```python
from build123d import *

# Parameters (mm, degrees)
Y_KSEKLIK_EKSTR_ZYON1_DEPTH = 3
RADYUS1_R                   = 0.5
KES_EKSTR_ZYON2_REACH       = 38.886
IZIM6_W                     = 13
IZIM6_H                     = 2.5


with BuildPart() as part:
    # Çizim1 → Yükseklik-Ekstrüzyon1 (new body)
    with BuildSketch(Plane.XY):
        Polygon((10, 21.25), (30, 21.25), (30, 6.25), (10, 6.25), (10, -18.75), (-10, -18.75), (-10, 21.25), align=None)
    extrude(amount=Y_KSEKLIK_EKSTR_ZYON1_DEPTH)

    # Radyus1
    radyus1_edges = [part.edges().sort_by_distance(p)[0] for p in [
        (-10, 21.25, 1.5),
        (30, 21.25, 1.5),
        (30, 6.25, 1.5),
        (10, -18.75, 1.5),
        (-10, -18.75, 1.5),
    ]]
    fillet(radyus1_edges, radius=RADYUS1_R)

    # Çizim6 → Kes-Ekstrüzyon2 (cut, up to next)
    with BuildSketch(Plane(origin=(0, 0, 0), x_dir=(-1, 0, 0), z_dir=(0, 0, -1)), mode=Mode.PRIVATE) as kes_ekstr_zyon2_sk1:
        with Locations((-17.130228212, 18)):
            Rectangle(IZIM6_W, IZIM6_H)
    kes_ekstr_zyon2_tool1 = extrude(kes_ekstr_zyon2_sk1.sketch, amount=-KES_EKSTR_ZYON2_REACH, mode=Mode.PRIVATE) & part.part
    add(kes_ekstr_zyon2_tool1.solids().sort_by_distance((17.130228, 18, 0))[0], mode=Mode.SUBTRACT)


solid = part.part
```
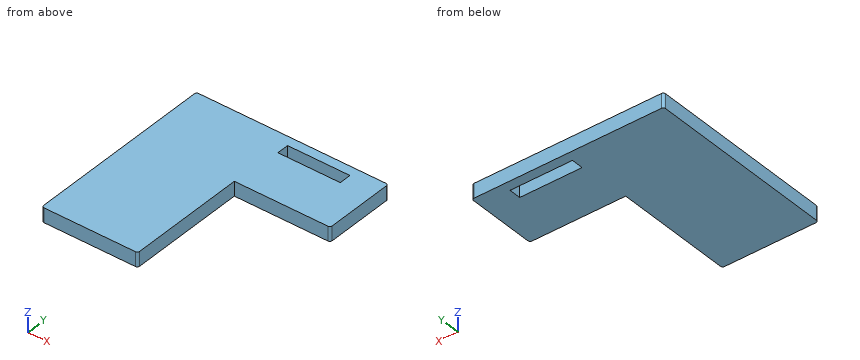
The model under review builds one solid part; all positions refer to its coordinate system, in mm. Give positions to 0.01 mm unless a question says otherwise; leave off trailing zeros. Write each loop counter-clockwise with the first axis right and the second up, starting at its lowest first coordinate (ties: lowest second). Pieces come first, ordered by that corner, then holes. Notation, with made-up numbers: M -16.5,30.25 L 31.5,30.25 A19 ccw 31.5,49.25 Z; hole C 70,23 d6. An arc over 180 degrees is marked long. Answer in a Markdown table with one row per item.
Item 1: Add section B-B on z = 2.2. Give the boundary of the cut face in (x, y).
Check sheet entries:
| item | result |
|---|---|
| outline | M -10,-18.25 A0.5 ccw -9.5,-18.75 L 9.5,-18.75 A0.5 ccw 10,-18.25 L 10,6.25 L 29.5,6.25 A0.5 ccw 30,6.75 L 30,20.75 A0.5 ccw 29.5,21.25 L -9.5,21.25 A0.5 ccw -10,20.75 Z; hole M 10.63,16.75 L 23.63,16.75 L 23.63,19.25 L 10.63,19.25 Z |
Item 2: Add section C-C on y = -1.5. Give the boundary of the cut face in (x, z).
Check sheet entries:
| item | result |
|---|---|
| outline | M -10,0 L 10,0 L 10,3 L -10,3 Z |
Item 3: For line 1 along Y through (x, z) = (18, 2.8); line 2 along X through (y, z) = (-10, 0.3); line 3 along Y through (x, z) = (27, 1.5), list the stretches that pass through material, from the lowest coordinate up.
Check sheet entries:
| item | result |
|---|---|
| line 1 | 6.25 to 16.75, 19.25 to 21.25 |
| line 2 | -10 to 10 |
| line 3 | 6.25 to 21.25 |
Item 4: For P1, Ø0.9, axis at y = -5.5, z = 2, coming from the +X side; P2, Ø1.5, axis at x = 15.5, z = 1, coming from the -Y side, all flat-tipped, find the tip position at first contact; note any pin that passes through.
Check sheet entries:
| item | result |
|---|---|
| P1 | x = 10 |
| P2 | y = 6.25 |
Item 5: Add section A-A on x = 23. Give the boundary of the cut face in (y, z), plus the area to 3 significant figures.
Check sheet entries:
| item | result |
|---|---|
| outline | M 6.25,0 L 16.75,0 L 16.75,3 L 6.25,3 Z; M 19.25,0 L 21.25,0 L 21.25,3 L 19.25,3 Z |
| area | 37.5 mm2 |
